```python
from build123d import *

# Parameters (mm, degrees)
PAD_DEPTH        = 7
HOLE_D           = 3.4
HOLE_CBORE_D     = 6
HOLE_CBORE_DEPTH = 3.4
CHAMFER_SIZE     = 0.2


with BuildPart() as part:
    # Sketch → Pad (new body)
    with BuildSketch(Plane.YZ):
        with BuildLine():
            Line((-2.5, 0), (-2.5, -0.8))
            Line((-2.5, -0.8), (7.25, -0.8))
            Line((7.25, 18.2), (7.25, -0.8))
            Line((-2.5, 18.2), (7.25, 18.2))
            Line((-2.5, 18.2), (-2.5, 17.4))
            Line((-2.5, 17.4), (-1.95, 17.4))
            ThreePointArc((-1.95, 17.4), (-1.4, 16.85), (-0.85, 17.4))
            Line((-0.85, 17.4), (0, 17.4))
            Line((0, 17.4), (0, 0))
            Line((0, 0), (-0.85, 0))
            ThreePointArc((-0.85, 0), (-1.4, 0.55), (-1.95, 0))
            Line((-1.95, 0), (-2.5, 0))
        make_face()
    extrude(amount=PAD_DEPTH)

    # Hole (through all)
    with Locations(Plane(origin=(0, 0, 0), x_dir=(0, 0, -1), z_dir=(0, -1, 0))):
        with Locations((-6.2, 3.5)):
            CounterBoreHole(HOLE_D / 2, HOLE_CBORE_D / 2, HOLE_CBORE_DEPTH)

    # Chamfer
    chamfer_edges = [part.edges().sort_by_distance(p)[0] for p in [
        (3.5, -2.5, 18.2),
        (3.5, -2.5, 17.4),
        (0, -2.5, 17.8),
        (7, -2.5, 17.8),
        (3.5, 7.25, 18.2),
        (0, 2.375, 18.2),
        (7, 2.375, 18.2),
        (3.5, -1.95, 17.4),
        (0, -2.225, 17.4),
        (7, -2.225, 17.4),
        (0, -1.4, 16.85),
        (0, -0.425, 17.4),
        (0, 0, 8.7),
        (0, -0.425, 0),
        (0, -1.4, 0.55),
        (0, -2.225, 0),
        (0, -2.5, -0.4),
        (0, 2.375, -0.8),
        (0, 7.25, 8.7),
        (7, -1.4, 16.85),
        (7, -0.425, 17.4),
        (7, 0, 8.7),
        (7, -0.425, 0),
        (7, -1.4, 0.55),
        (7, -2.225, 0),
        (7, -2.5, -0.4),
        (7, 2.375, -0.8),
        (7, 7.25, 8.7),
        (3.5, 7.25, -0.8),
        (1.8, 7.25, 6.2),
        (3.5, -0.85, 17.4),
        (3.5, 0, 17.4),
        (3.5, 0, 0),
        (0.5, 0, 6.2),
        (3.5, -0.85, 0),
        (3.5, -1.95, 0),
        (3.5, -2.5, 0),
        (3.5, -2.5, -0.8),
        (5.2, 5.325, 6.2),
        (1.8, 3.4, 6.2),
        (0.5, 3.4, 6.2),
        (6.5, 1.7, 6.2),
    ]]
    chamfer(chamfer_edges, length=CHAMFER_SIZE)


solid = part.part
```
Could you check a few things on this model? Use its own coordinates, in mm. A direction names the side the tool comes from. Round coordinates to 2 decimals unless told otherwise and drop trailing zeros. Loops run counter-clockwise (first coordinate to the right, second up) from the corner with the lowest first, then second, coordinate; pieces in that order, holes last. Notation, with made-up numbers: M 43.5,80 L 80.5,80 A11 cw 80.5,99 Z; hole C 49,32 d4. An arc over 180 degrees is marked long. Write item = value, one per line.
1. I want a section at A-A, the plane z = 6.2. Write out the boundary of the cut face in (x, y).
Results below:
outline = M 0,0.2 L 0.2,0 L 0.3,0 L 0.5,0.2 L 0.5,3.2 L 0.7,3.4 L 1.6,3.4 L 1.8,3.6 L 1.8,7.05 L 1.6,7.25 L 0.2,7.25 L 0,7.05 Z; M 5.2,3.6 L 5.4,3.4 L 6.3,3.4 L 6.5,3.2 L 6.5,0.2 L 6.7,0 L 6.8,0 L 7,0.2 L 7,7.05 L 6.8,7.25 L 5.4,7.25 L 5.2,7.05 Z
2. Thinking about a two-plate mould opening in Y: for faces 1 (the face through (3.45, -1.39, 0.55)), 2 (the face through (0, 3, 9)), 3 (the face through (3, 3.4, 4)), which applies, +Y half, -Y half, draft (parallel to the pull), parting line (faces both ways), or undercut?
Results below:
face_1 = undercut
face_2 = draft
face_3 = -Y half
3. I want a section at C-C, the plane z = 1.75. Write out the boundary of the cut face in (x, y).
Results below:
outline = M 0,0.2 L 0.2,0 L 6.8,0 L 7,0.2 L 7,7.05 L 6.8,7.25 L 0.2,7.25 L 0,7.05 Z
4. I want a section at D-D, the plane y = 5. Write out the boundary of the cut face in (x, z).
Results below:
outline = M 0,-0.6 L 0.2,-0.8 L 6.8,-0.8 L 7,-0.6 L 7,18 L 6.8,18.2 L 0.2,18.2 L 0,18 Z; hole C 3.5,6.2 d3.4
5. I want a section at B-B, the plane y = 1.25. Write out the boundary of the cut face in (x, z).
Results below:
outline = M 0,-0.6 L 0.2,-0.8 L 6.8,-0.8 L 7,-0.6 L 7,18 L 6.8,18.2 L 0.2,18.2 L 0,18 Z; hole C 3.5,6.2 d6
6. Which directions (+Z, -Z, +X, -X, +Y, -Y) give clear straight access to the entire face, cutting with the end or side of a thin tool? Please do faces 4 (the face through (3.45, -1.41, 16.85)), 5 (the face through (2.85, 5.35, 7.77)), 6 (the face through (4.4, 1.68, 3.34)).
Results below:
face_4 = +X, -X
face_5 = +Y, -Y
face_6 = -Y
7. I need wall thicknesses on probe 1 along X at (y, z) = (2.4, 6.2); probe 2 along Y at (x, z) = (3.5, 11.5); probe 3 along Z at (x, y) = (1, 0.5). Which ranges of each line are inside material? Lowest first, please.
Results below:
probe_1 = 0 to 0.5, 6.5 to 7
probe_2 = 0 to 7.25
probe_3 = -0.8 to 4.54, 7.86 to 18.2
